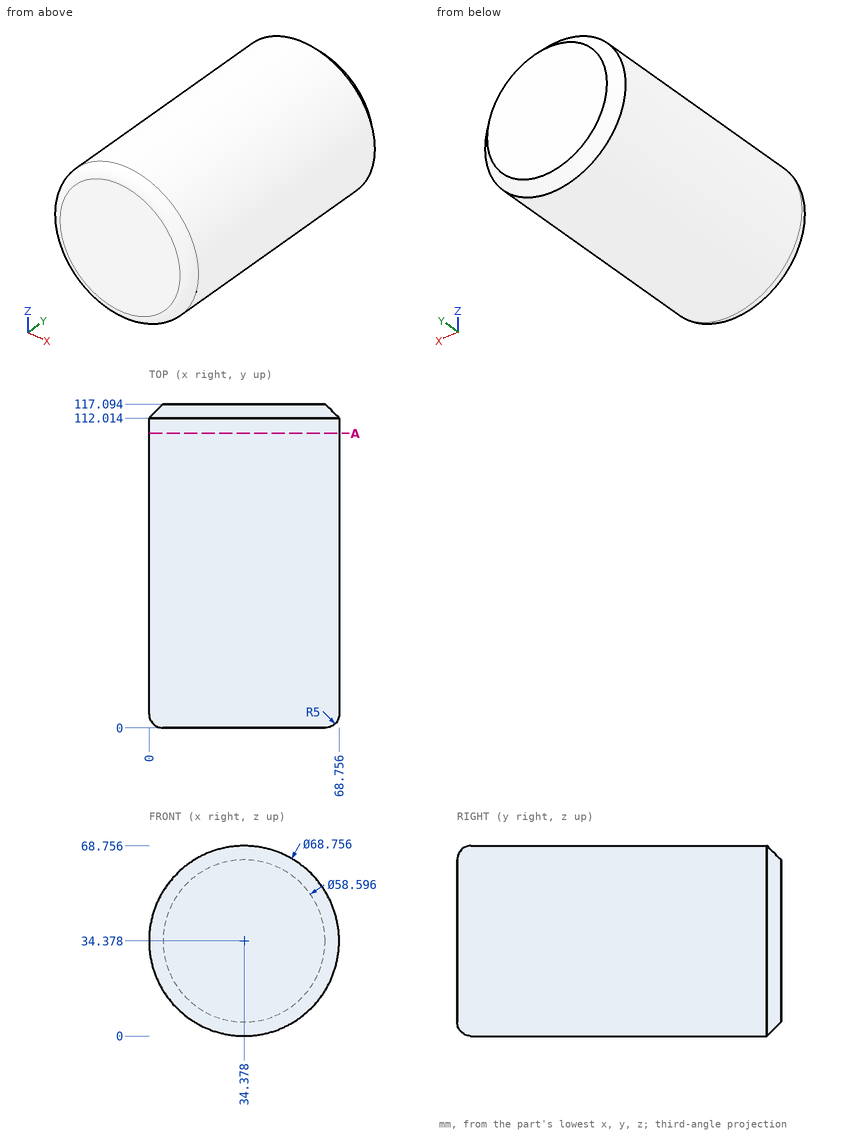
Source: three-view drawing plus pictorial views. Frame: mm from the lowest corner of the part. Give positions to 0.01 mm unless a question says otherwise; leave off trailing zeros. Loops run counter-clockwise (first coordinate to the right, second up) from the corner with the lowest first, then second, coordinate; pieces in that order, holes last. Notation, with made-up numbers: (-5.5, 64) -> (12.5, 64) arc R14 ccw to (12.5, 75) -> close; hole circle Ø10 at (-31, -35.5). An arc over 180 degrees is marked (long way). Put each result on its own line as item: value. Start each with the question number.
1) Material intervals for probe 1 along Z at (x, y) = (33, 107.5); probe 2 along X at (y, z) = (23.5, 23); probe 3 along X at (y, z) = (108.5, 55) (1 decimal), sorted ascending.
2) Contact query for flat-ended pins moving along their axis: P1, Ø4, axis at y = 72, z = 62, coming from the -X side; P2, Ø2, axis at y = 48, z = 13.5, coming from the +X side (1 decimal); P3, Ø5, axis at y = 91, z = 27.5, coming from the -X side. Output: stop coordinate, or through.
3) Cut plane A-A (y = 106.5). Return loops of the section in (x, z) (1 decimal).
Results are:
1. probe 1: z = 0.03 to 68.73
1. probe 2: x = 1.94 to 66.82
1. probe 3: x = 6.9 to 61.9
2. P1: stops at x = 11.46
2. P2: stops at x = 62.4
2. P3: stops at x = 0.28
3. outline: circle Ø68.8 at (34.4, 34.4)
